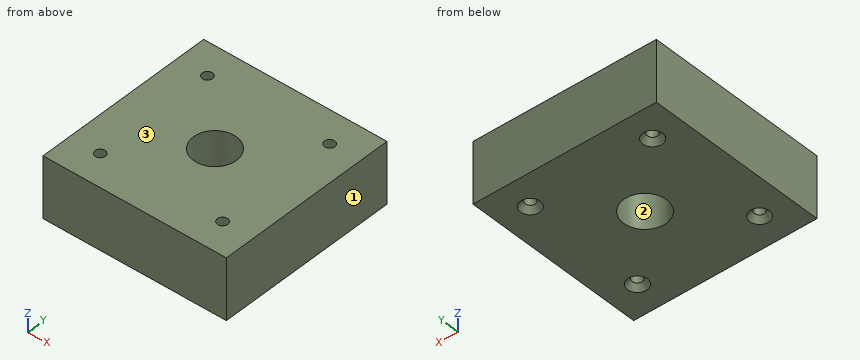
Autodesk Inventor part; units mm, degrees
ref_plane "YZ Plane" through (0, 0, 0) normal (1, 0, 0) x (0, 1, 0)
ref_plane "XZ Plane" through (0, 0, 0) normal (0, 1, 0) x (-1, 0, 0)
ref_plane "XY Plane" through (0, 0, 0) normal (0, 0, 1) x (1, 0, 0)
sketch "Sketch1" plane through (0, 0, 0) normal (0, 0, 1) x (1, 0, 0)
  line L0 (0, 0) -> (150, 0)
  line L1 (150, 0) -> (150, 150)
  line L2 (150, 150) -> (0, 150)
  line L3 (0, 150) -> (0, 0)
  dimension "d0" = 150
  dimension "d1" = 150
extrude "Extrusion1" add sketch "Sketch1" along normal blind 50
sketch "Sketch2" plane through (0, 0, 50) normal (0, 0, 1) x (1, 0, 0)
  line L0 (150, 0) -> (150, 150)
  line L1 (150, 150) -> (0, 150)
  point P0 (0, 0)
  point P1 (75, 75)
  point P2 (150, 75)
  point P3 (75, 150)
hole "Hole1" at (75, 75, 50) direction (0, 0, -1) diameter 35 end through all
sketch "Sketch3" plane through (0, 0, 0) normal (0, 0, -1) x (-1, 0, 0)
  line L0 (-150, 150) -> (0, 150)
  line L1 (0, 150) -> (0, 0)
  line L2 (0, 0) -> (-150, 0)
  line L3 (-150, 0) -> (-150, 150)
  point P0 (-125, 125)
  point P1 (-25, 125)
  point P2 (-25, 25)
  point P3 (-125, 25)
  dimension "d11" = 25
  dimension "d12" = 25
  dimension "d13" = 25
  dimension "d14" = 25
hole "Hole2" at (125, 125, 0) at (25, 125, 0) at (25, 25, 0) at (125, 25, 0) direction (0, 0, 1) diameter 8.433 end through all countersink diameter 16.129 countersink angle 82
properties part number "Top_Spacer" material "Wood (Birch)"
Input: part model. Units: mm. Frame: model coordinates. Face numbers are marked on the shaded views. Coordinates: 2 decimals unless noted, no trailing zeros. Write each loop counter-clockwise with the first axis right and the second up, starting at its lowest first coordinate (ties: lowest second). Pieces come first, ordered by that corner, then holes. Notation, with made-up numbers: M 44.5,1 L 49.5,1 A23 cw 49.5,11 Z; hole C 76,37 d5. An arc over 180 degrees is marked long. Answer as a JSON object with one key per item and string values. Group by question number.
(1) Section D-D on z = 30.5. Output: boundary loops of the cut face in (x, y), plus the area to 3 significant figures.
(2) Ray query, line 1 along X through (y, z) = (25, 40.5); line 2 along Y through (x, z) = (75, 47). Return the intervals inside material, ascending. Write a range as [from, to].
(3) Section B-B on y = 75. Output: boundary loops of the cut face in (x, z).
(4) Contact query for flat-ended pins moving along their axis: P1, Ø11, axis at x = 125, y = 125, coming from the -Z side; P2, Ø13.5, axis at x = 25, y = 125, coming from the -Z side; P3, Ø7.5, axis at x = 25, y = 25, coming from the -Z side. Output: stop coordinate, or through.
(5) Section A-A on x = 25. Output: boundary loops of the cut face in (y, z).
(6) Mould query, pull axis X, two halves, no side actions, for the marked faces 1, 2 and 3. Classes: pulls with the +X half, pulls with the -X half, needs draft (parallel to the pull), parting line crosses it, or undercut.
Result set:
{
 "1": {"outline": "M 0,0 L 150,0 L 150,150 L 0,150 Z; hole C 25,25 d8.43; hole C 25,125 d8.43; hole C 75,75 d35; hole C 125,25 d8.43; hole C 125,125 d8.43", "area": "21,300 mm2"},
 "2": {"line 1": "x = [0, 20.78], [29.22, 120.78], [129.22, 150]", "line 2": "y = [0, 57.5], [92.5, 150]"},
 "3": {"outline": "M 0,0 L 57.5,0 L 57.5,50 L 0,50 Z; M 92.5,0 L 150,0 L 150,50 L 92.5,50 Z"},
 "4": {"P1": "stops at z = 2.95", "P2": "stops at z = 1.51", "P3": "passes through"},
 "5": {"outline": "M 0,0 L 16.94,0 L 20.78,4.43 L 20.78,50 L 0,50 Z; M 29.22,4.43 L 33.06,0 L 116.94,0 L 120.78,4.43 L 120.78,50 L 29.22,50 Z; M 129.22,4.43 L 133.06,0 L 150,0 L 150,50 L 129.22,50 Z"},
 "6": {"face 1": "pulls with the +X half", "face 2": "undercut", "face 3": "needs draft"}
}
